Autodesk Inventor part; units mm, degrees
ref_plane "Work Plane1" through (29, 0, 0) normal (0, -1, 0) x (1, 0, 0)
ref_plane "YZ Plane" through (0, 0, 0) normal (1, 0, 0) x (0, 1, 0)
ref_plane "XZ Plane" through (0, 0, 0) normal (0, 1, 0) x (-1, 0, 0)
sketch "Sketch1" plane through (0, 0, 0) normal (0, 0, 1) x (1, 0, 0)
  line L0 (-0.0667, 0) -> (10, 0)
  line L1 (10, 0) -> (10, 2)
  line L2 (10, 2) -> (2.1, 2)
  line L3 (2.1, 2) -> (1.6705, 2)
  line L4 (1.6705, 2) -> (0, 2)
  line L5 (0, 2) -> (0, 3.8)
  line L6 (0, 3.8) -> (-2.2, 3.8)
  line L7 (-2.2, 3.8) -> (-2.2, 1.4434)
  line L8 (-2.2, 1.4434) -> (-0.9, 1.4434)
  line L9 (-0.9, 1.4434) -> (-0.0667, 0)
  line L10 (-4.64, 0) -> (12.44, 0)
  line L11 (0, -0.76) -> (0, 4.56)
  line L12 (2.1, 2) -> (0, 2) construction
  dimension "d1" = 7.9
  dimension "d2" = 0.4295
  dimension "d3" = 2.2
  dimension "d4" = 1.3
  dimension "d5" = 60
  dimension "d6" = 4
  dimension "d7" = 4
  dimension "d8" = 2.8868
  dimension "d9" = 7.6
  dimension "d26" = 10
revolve "Body" add sketch "Sketch1" angle 360 about axis through (-0.0667, 0, 0) along (1, 0, 0)
sketch "Sketch2" plane through (-2.2, 0, 0) normal (-1, 0, 0) x (0, 0, 1)
  circle A0 centre (0, 0) radius 1.4434
  line L0 (0, -5.32) -> (0, 5.32)
  line L1 (-5.32, 0) -> (5.32, 0)
  line L2 (1.4434, 0) -> (0.7217, -1.25)
  line L3 (0.7217, -1.25) -> (-0.7217, -1.25)
  line L4 (-0.7217, -1.25) -> (-1.4434, 0)
  line L5 (-1.4434, 0) -> (-0.7217, 1.25)
  line L6 (-0.7217, 1.25) -> (0.7217, 1.25)
  line L7 (0.7217, 1.25) -> (1.4434, 0)
extrude "Slot" add sketch "Sketch2" against normal up to next contours L7 A0 | A0 L2 | L6 L0 A0 | A0 L0 L3 | L0 L6 A0 | A0 L3 L0 | L4 A0 | A0 L5
fillet "Fillet1" radius 1.9 1 edges at (-2.2, -3.8, 0)
thread "Thread"
chamfer "Chamfer1" distance 0.4294 distance2 0.4294 1 edges at (10, -2, 0) measured on face at (10, 0.556, 0.0273)
ref_plane "Work Plane1" through (29, 0, 0) normal (0, -1, 0) x (1, 0, 0)
fillet "Fillet2" radius 0.4 1 edges at (0, -2, 0)
equation "\"d30\" = R"
equation "\"d17\" = RR"
equation "\"d13\" = GEL"
equation "\"d15\" = -0.5 * SPD + 0.5 * GD"
equation "\"d16\" = GUL"
equation "\"d1\" = GEL"
equation "\"d3\" = KOH"
equation "\"d4\" = INTI"
equation "\"d6\" = GD"
equation "\"d7\" = BDM"
equation "\"d8\" = 1.1547 * SW"
equation "\"d9\" = KOD"
equation "\"d26\" = NLG"
equation "\"GD\" = NND"
equation "\"NLG\" = 10"
equation "\"GEL\" = 7.9"
equation "\"KOD\" = 7.6"
equation "\"KOH\" = 2.2"
equation "\"INTI\" = 1.3"
equation "\"GAL\" = 0.61345 * PTC"
equation "\"GUL\" = 0.61345 * PTC"
equation "\"BDM\" = NND"
equation "\"SW\" = 2.5"
equation "\"RR\" = 1.9"
equation "\"SPD\" = NND - 1.2269 * PTC"
equation "\"R\" = 0.4"
equation "\"TOA\" = 30deg"
equation "\"GD1\" = THREADDIA - 1.2269 * PTC"
equation "\"THREADDIA\" = 4"
equation "\"PTC\" = 0.7"
equation "\"NND\" = 4"
equation "\"KOH1\" = 0.3"
equation "\"E0\" = 2.873"
properties part number "ISO 7380-1 - M4 x 10" material "Steel"
Work out the finished part from the listing and answer in its coordinate system (mm). A direction names the side the tool comes from. Round coordinates to 2 decimals unless told otherwise and drop trailing zeros. Write each loop counter-clockwise with the first axis right and the second up, starting at its lowest first coordinate (ties: lowest second). Pieces come first, ordered by that corner, then holes. Notation, with made-up numbers: (89, -20) - (114, -20) arc R8 ccw to (114, -6) - close; hole circle Ø8 at (85, -11.5). An arc over 180 degrees is marked (long way). Return JSON: item names as keys, results as strings. Group by question number.
Q1. Each of these flat-tipped pins is pushed along its axis until it touches: pin 1 Ø0.7 at (x, z) = (-1.5, 0.5) entering from +Y; pin 2 Ø1.1 at (x, z) = (-1.5, 0) entering from -Y. Where does it stop, or does it pass through?
Q2. Find the intervals of material crossed by L1, parallel to X at y = 1, z = 2.75; L2, parallel to X at y = -1, z = 1.5; L3, parallel to Z at x = 7.25, y = 1.75, in increasing order.
Q3. For faces 1 (the cylindrical face through (5, 0, 2)), 2 (the flat face through (-1.504, -0.616, 1.088)), determine the directions among +Z, -Z, +X, -X, +Y, -Y from which every point of the face is accessible in a straight line to the end or side of a thin tool.
Q4. The mould has two halves that part along Y. Classify faces 3 (the flat face through (10, 0, 0)), 4 (the cylindrical face through (-0.15, -2.8, -2.57)), 5 (the flat face through (-1.5, 0.63, 1.08)): released by +Y, released by -Y, zero draft, split by the parting line, or undercut.
Q5. The part is cut by section A-A on x = 9. Write down the section's boundary in (y, z).
Solved:
{
 "1": {"pin 1": "y = 3.57", "pin 2": "y = -3.69"},
 "2": {"L1": "-1.9 to 0", "L2": "-2.2 to 9.77", "L3": "-0.97 to 0.97"},
 "3": {"face 1": "+X", "face 2": "-X"},
 "4": {"face 3": "zero draft", "face 4": "split by the parting line", "face 5": "undercut"},
 "5": {"outline": "circle Ø4 at (0, 0)"}
}
